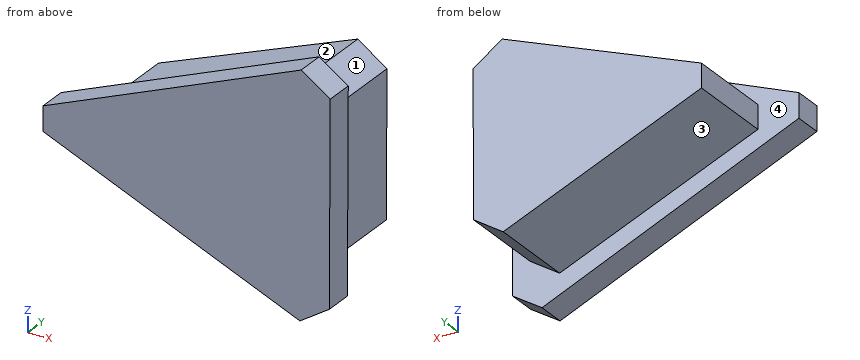
Autodesk Inventor part; units mm, degrees
ref_plane "YZ Plane" through (0, 0, 0) normal (1, 0, 0) x (0, 1, 0)
ref_plane "XZ Plane" through (0, 0, 0) normal (0, 1, 0) x (-1, 0, 0)
ref_plane "XY Plane" through (0, 0, 0) normal (0, 0, 1) x (1, 0, 0)
sketch "Náčrt1" plane through (0, 0, 0) normal (0, 1, 0) x (-1, 0, 0)
  line L0 (-9, 0.0297) -> (-8.9669, -7.4702)
  line L1 (-8.9669, -7.4702) -> (-0.0106, -3.7456)
  line L2 (-9, 0.0297) -> (-0.0106, -3.7456)
  point P0 (0, 0)
  dimension "d1" = 7.5
  dimension "d23" = 9.7
  dimension "d24" = 9.75
extrude "Vysunutí1" add sketch "Náčrt1" along normal blind 0.8
sketch "Náčrt2" plane through (0, 0.8, 0) normal (0, 1, 0) x (1, 0, 0)
  line L0 (8.4965, 0.7703) -> (8.4705, 6.6703)
  line L1 (9, -0.0297) -> (8.9669, 7.4702)
  line L2 (8.4705, 6.6703) -> (1.1705, 3.7203)
  line L3 (8.4965, 0.7703) -> (1.1705, 3.7203)
  point P0 (0, 0)
  dimension "d6" = 0.5
  dimension "d16" = 5.9
  dimension "d17" = 0.8
  dimension "d18" = 2.95
extrude "Vysunutí2" add sketch "Náčrt2" along normal blind 2.5
chamfer "Zkosení1" distance 0.9 angle 45 3 edges at (1.1705, 2.05, -3.7203) (8.4965, 2.05, -0.7703) (8.4705, 2.05, -6.6703)
chamfer "Zkosení2" distance 0.9 angle 45 3 edges at (9, 0.4, 0.0297) (8.9669, 0.4, -7.4702) (0.0106, 0.4, -3.7456)
properties part number "SideButton"
Source: CAD feature listing. Evaluate the final solid. Frame: model axes, mm. Face numbers are marked on the shaded views. A direction names the side the tool comes from. Give positions to 0.01 mm unless a question says otherwise; leave off trailing zeros. Order: outer loops, then holes, each group sorted by start corner. A loop starts at its lowest first (then second) coordinate and runs counter-clockwise, first axis right, second up. Notation, with made-up numbers: (-31, 19.5) -> (-6, 19.5) arc R29 cw to (-6, 54.5) -> close; hole circle Ø4 at (-14, -4). An arc over 180 degrees is marked (long way). Use a Markdown table: item, result.
Q1. Section D-D (y = 0.3). Return the cut outline in (x, z).
A:
| item | result |
|---|---|
| outline | (0.84, -4.09) -> (8.14, -7.12) -> (8.97, -6.57) -> (9, -0.87) -> (8.17, -0.32) -> (0.84, -3.4) -> close |
Q2. Material intervals for line 1 (Y direction, x = 8.5, z = -1.5); line 2 (Z direction, x = 3.25, y = 2.45); line 3 (Z direction, x = 1.25, y = 0.7), sorted ascending. Write a range as [from, to].
A:
| item | result |
|---|---|
| line 1 | [0, 0.8] |
| line 2 | [-4.56, -2.88] |
| line 3 | [-4.26, -3.23] |
Q3. First-contact query: P1, Ø1.5, axis at x = 4.5, y = 1, coming from the -Z side; P2, Ø1, axis at y = 2, z = -3, coming from the -X side. Flat tips, straight axial feed; report the tip coordinate or a pass-through.
A:
| item | result |
|---|---|
| P1 | z = -5.91 |
| P2 | x = 2.01 |
Q4. Section B-B (x = 8). Return the cut outline in (y, z), and give its area (3 significant figures).
A:
| item | result |
|---|---|
| outline | (0, -7.07) -> (0.8, -7.07) -> (0.8, -6.09) -> (3.3, -6.09) -> (3.3, -1.34) -> (0.8, -1.34) -> (0.8, -0.39) -> (0, -0.39) -> close |
| area | 17.2 mm^2 |
Q5. Section A-A (y = 3). Return the cut outline in (x, z), and give its area (3 significant figures).
A:
| item | result |
|---|---|
| outline | (2, -4.06) -> (7.64, -6.33) -> (8.47, -5.77) -> (8.49, -1.67) -> (7.66, -1.11) -> (2.01, -3.38) -> close |
| area | 20.5 mm^2 |
Q6. Access query for the marked faces 1, 2, 3 and 4. Directions: +Z, -Z, +X, -X, +Y, -Y. A direction counts if a zero-diameter tool reaches every point of the face in a straight line with its end or side. Return the directions, or none.
A:
| item | result |
|---|---|
| face 1 | +Z, +X, +Y |
| face 2 | +Z, -X, +Y |
| face 3 | -Z, -X, +Y |
| face 4 | +Y |
Q7. Section C-C (z = -2.25). Return the cut outline in (x, y).
A:
| item | result |
|---|---|
| outline | (3.57, 0) -> (8.99, 0) -> (8.99, 0.8) -> (8.49, 0.8) -> (8.49, 3.3) -> (4.82, 3.3) -> (4.82, 0.8) -> (3.57, 0.8) -> close |
